from build123d import *

# Parameters (mm, degrees)
F0_R     = 61.338587
F1_DEPTH = 19.05
F2_R     = 54.988587
F3_DEPTH = 6.35
F4_R     = 54.988587
F5_DEPTH = 6.35
F6_R     = 15.875
F7_DEPTH = 12.701


with BuildPart() as f1:
    # F0 (on Top) → F1 (new body)
    with BuildSketch(Plane.XY):
        Circle(F0_R)
    extrude(amount=F1_DEPTH)

    # F2 (on face) → F3 (cut)
    with BuildSketch(Plane(origin=(0, 0, 0), x_dir=(1, 0, 0), z_dir=(0, 0, -1))):
        Circle(F2_R)
    extrude(amount=-F3_DEPTH, mode=Mode.SUBTRACT)

    # F4 (on face) → F5 (cut)
    with BuildSketch(Plane.XY.offset(19.05)):
        Circle(F4_R)
    extrude(amount=-F5_DEPTH, mode=Mode.SUBTRACT)

    # F6 (on face) → F7 (cut, through all)
    with BuildSketch(Plane.XY.offset(12.7)):
        Circle(F6_R)
    extrude(amount=-F7_DEPTH, mode=Mode.SUBTRACT)


solid = f1.part
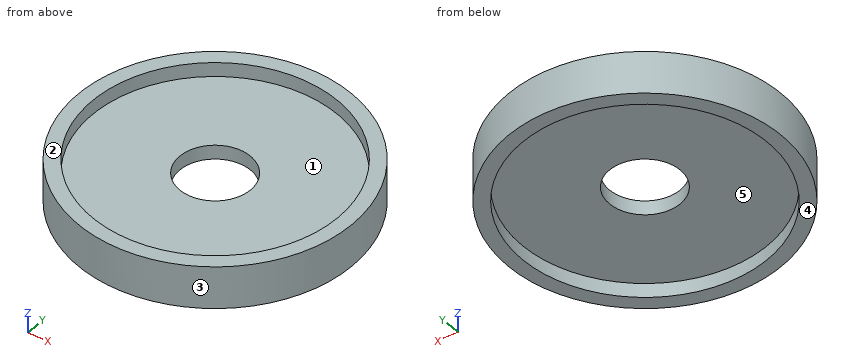
Build history of the part. All positions in model axes, mm. Face numbers are marked on the shaded views. A direction names the side the tool comes from. Give positions to 0.01 mm unless a question says otherwise; leave off trailing zeros. Order: outer loops, then holes, each group sorted by start corner. A loop starts at its lowest first (then second) coordinate and runs counter-clockwise, first axis right, second up. Notation, with made-up numbers: M 11.5,55.25 L 68.5,55.25 A10 ccw 68.5,72.25 Z; hole C 11.5,78 d3. An arc over 180 degrees is marked long. Use one line per item in the form item = value.
1) Two-plate mould, pull along X, no slides. Class the marked faces 1, 2 and 3: released by +X, released by -X, zero draft, split by the parting line, or undercut.
Calculated:
face_1 = undercut
face_2 = zero draft
face_3 = split by the parting line
2) Saw through at D-D (x = -43). Give the cut face in (y, z), plus the area to 3 significant figures.
Calculated:
outline = M -43.74,0 L -34.27,0 L -34.27,6.35 L 34.27,6.35 L 34.27,0 L 43.74,0 L 43.74,19.05 L 34.27,19.05 L 34.27,12.7 L -34.27,12.7 L -34.27,19.05 L -43.74,19.05 Z
area = 796 mm2
3) Saw through at A-A (x = 0). Give the cut face in (y, z) (3 decimals), plus the area to 3 significant figures.
Calculated:
outline = M -61.339,0 L -54.989,0 L -54.989,6.35 L -15.875,6.35 L -15.875,12.7 L -54.989,12.7 L -54.989,19.05 L -61.339,19.05 Z; M 15.875,6.35 L 54.989,6.35 L 54.989,0 L 61.339,0 L 61.339,19.05 L 54.989,19.05 L 54.989,12.7 L 15.875,12.7 Z
area = 739 mm2
4) Drop flat-ended pins along their axis: pin 1 (10 mm diameter, centred on x = -7.5, z = 4.5, fed in from +Y); pin 2 (8 mm diameter, centred on y = 19, z = 14.5, fed in from +X); pin 3 (1.5 mm diameter, centred on y = 31.5, z = 2, fed in from -X). Give the stop position or say it passes through.
Calculated:
pin_1 = 61.29
pin_2 = 59.48
pin_3 = -53.07
5) Probe probe 1 along Y at (x, z) = (0, 11) (3 decimals); probe 2 along Y at (x, z) = (0, 2.5); probe 3 along Z at (x, y) = (-27, -41.5). List the from-to ranges inside material, lowest first.
Calculated:
probe_1 = -61.339 to -15.875, 15.875 to 61.339
probe_2 = -61.34 to -54.99, 54.99 to 61.34
probe_3 = 6.35 to 12.7
6) Saw through at C-C (z = 2.75). Give the cut face in (x, y), plus the area to 3 significant figures.
Calculated:
outline = C 0,0 d122.68; hole C 0,0 d109.98
area = 2,320 mm2
7) Tool access for the marked faces 4 and 5: list every direction of +Z, -Z, +X, -X, +Y, -Y with a clear straight run to the whole face (end or side of a thin tool).
Calculated:
face_4 = -Z, +X, -X, +Y, -Y
face_5 = -Z
